Autodesk Inventor part; units mm, degrees
ref_plane "YZ Plane" through (0, 0, 0) normal (1, 0, 0) x (0, 1, 0)
ref_plane "XZ Plane" through (0, 0, 0) normal (0, 1, 0) x (-1, 0, 0)
ref_plane "XY Plane" through (0, 0, 0) normal (0, 0, 1) x (1, 0, 0)
sketch "Sketch2" plane through (0, 0, 0) normal (0, 0, 1) x (1, 0, 0)
  line L0 (25, 8) -> (25, 0)
  line L1 (25, 0) -> (-25, 0)
  line L2 (-25, 0) -> (-25, 8)
  line L3 (0, -7) -> (0, 42)
  arc A0 (15, 20) -> (-15, 20) centre (0, 20) ccw
  line L4 (0, 42) -> (0, -7)
  line L5 (-15, 20) -> (-15, 8)
  line L6 (15, 20) -> (15, 8)
  line L7 (-35, 0) -> (35, 0)
  line L8 (-25, 8) -> (-15, 8)
  line L9 (15, 8) -> (25, 8)
  point P0 (0, 0)
  dimension "d4" = 50
  dimension "d6" = 20
  dimension "d7" = 30
  dimension "d8" = 8
  dimension "d9" = 8
extrude "Extrusion2" add sketch "Sketch2" against normal blind 10
sketch "Sketch3" plane through (0, 0, 0) normal (0, 0, 1) x (1, 0, 0)
  arc A0 (15, 20) -> (-15, 20) centre (0, 20) ccw
  circle A1 centre (0, 20) radius 13.05
  point P0 (0, 0)
  dimension "d12" = 26.1
extrude "Extrusion3" cut sketch "Sketch3" against normal blind 8
sketch "Sketch4" plane through (0, 20, -8) normal (0, 0, 1) x (1, 0, 0)
  circle A0 centre (0, 0) radius 6.05
  point P0 (0, -20)
  dimension "d15" = 12.1
extrude "Extrusion4" cut sketch "Sketch4" against normal blind 1
sketch "Sketch5" plane through (0, 20, -9) normal (0, 0, 1) x (1, 0, 0)
  circle A0 centre (0, 0) radius 1.75
  point P0 (0, -20)
  dimension "d18" = 3.5
extrude "Extrusion5" cut sketch "Sketch5" against normal blind 1
sketch "Sketch6" plane through (-25, 0, 0) normal (0, -1, 0) x (1, 0, 0)
  circle A0 centre (5, -5) radius 2
  circle A1 centre (45, -5) radius 2
  line L0 (25, -12) -> (25, 2)
  line L1 (50, -10) -> (0, -10)
  point P0 (25, 0)
  dimension "d21" = 4
  dimension "d22" = 40
  dimension "d23" = 5
extrude "Extrusion6" cut sketch "Sketch6" against normal blind 6
fillet "Fillet1" radius 1 4 edges at (-15, 8, -5) (-25, 8, -5) (15, 8, -5) (25, 8, -5)
properties part number "sg_motor_mount"
Read the model definition and answer for the solid it produces. Units are mm, in the model's axes. A direction names the side the tool comes from. Give positions to 0.01 mm unless a question says otherwise; leave off trailing zeros. Write each loop counter-clockwise with the first axis right and the second up, starting at its lowest first coordinate (ties: lowest second). Pieces come first, ordered by that corner, then holes. Notation, with made-up numbers: (-0.5, 69) -> (20.5, 69) arc R38 cw to (20.5, 108) -> close; hole circle Ø5 at (-27.75, 9). An arc over 180 degrees is marked (long way). Answer as a JSON object with one key per item and string values. Group by question number.
1) Each of these flat-tipped pins is pushed along its axis until it touches: P1, Ø4, axis at x = -18.5, z = -4.5, coming from the +Y side; P2, Ø3, axis at y = 16.5, z = -7, coming from the +X side; P3, Ø1.5, axis at x = 4, z = -3.5, coming from the +Y side. Where does it stop, or does it pass through?
2) Consider L1, parallel to Z at x = 20, y = 3.3; L2, parallel to Y at x = 0, z = -8.5; L3, parallel to Z at x = 5.5, y = 10. Determine where each line is inside the solid, lowest interval first. Write a range as from..to.
3) Find section B-B (z = -2.5). Write down the section's boundary in (x, y).
4) The mould has two halves that part along X. Classify faces 1 (the cylindrical face through (0, 35, -5)), 2 (the cylindrical face through (-2.83, 7.26, -3.94)), 3 (the flat face through (0, 14, -10)): +X half, -X half, draft (parallel to the pull), parting line (faces both ways), or undercut.
5) Find section D-D (y = 27). Write down the section's boundary in (x, z), and give its area (3 significant figures).
6) A tool of negligible diameter and unlimited length cuts with its end or side. For faces 4 (the cylindrical face through (-21.6, 3, -6.2)), 5 (the flat face through (20, 8, -5)), 6 (the flat face through (-20, 8, -5)), from which of +Z, -Z, +X, -X, +Y, -Y can it reach the whole face along a straight path? Write none if from no direction.
7) Find section C-C (x = 20). Write down the section's boundary in (y, z).
8) Find section A-A (x = 0). Write down the section's boundary in (y, z).
Values follow:
{
 "1": {"P1": "stops at y = 8", "P2": "stops at x = 15", "P3": "stops at y = 34.64"},
 "2": {"L1": "z = -10..-7, -3..0", "L2": "y = 0..13.95, 26.05..35", "L3": "z = -10..-8"},
 "3": {"outline": "(-25, 0) -> (25, 0) -> (25, 7) arc R1 ccw to (24, 8) -> (16, 8) arc R1 cw to (15, 9) -> (15, 20) arc R15 ccw to (-15, 20) -> (-15, 9) arc R1 cw to (-16, 8) -> (-24, 8) arc R1 ccw to (-25, 7) -> close; hole circle Ø26.1 at (0, 20)"},
 "4": {"face 1": "parting line", "face 2": "undercut", "face 3": "draft"},
 "5": {"outline": "(-13.27, -10) -> (13.27, -10) -> (13.27, 0) -> (11.01, 0) -> (11.01, -8) -> (-11.01, -8) -> (-11.01, 0) -> (-13.27, 0) -> close", "area": "89.1 mm2"},
 "6": {"face 4": "-Y", "face 5": "+Z, -Z, +X, +Y", "face 6": "+Z, -Z, -X, +Y"},
 "7": {"outline": "(0, -10) -> (8, -10) -> (8, 0) -> (0, 0) -> (0, -3) -> (6, -3) -> (6, -7) -> (0, -7) -> close"},
 "8": {"outline": "(0, -10) -> (18.25, -10) -> (18.25, -9) -> (13.95, -9) -> (13.95, -8) -> (6.95, -8) -> (6.95, 0) -> (0, 0) -> close; (21.75, -10) -> (35, -10) -> (35, 0) -> (33.05, 0) -> (33.05, -8) -> (26.05, -8) -> (26.05, -9) -> (21.75, -9) -> close"}
}
